from build123d import *

# Parameters (mm, degrees)
F0_R     = 74.8
F0_R_2   = 3.5
F0_R_3   = 26
F1_DEPTH = 7.9
F2_DEPTH = 7.9
F3_R     = 66.1
F3_R_2   = 3.5
F3_R_3   = 26
F4_DEPTH = 2
F8_DEPTH = 5.9
F9_DEPTH = 2


# Not quite as in the source:
# - a feature names something its author has since deleted; it is built from what else it names


with BuildPart() as f1:
    # F0 (on Front) → F1 (new body)
    with BuildSketch(Plane.XZ):
        Circle(F0_R)
        with BuildLine():
            ThreePointArc((-23.816128087, -54.7983078474), (-42.2496301759, -42.2496301759), (-54.7983078474, -23.816128087))
            ThreePointArc((-54.7983078474, -23.816128087), (-54.50218665, -19.353932752), (-51.1097752784, -22.2677652896))
            ThreePointArc((-51.1097752784, -22.2677652896), (-39.4212030512, -39.4212030512), (-22.2677652896, -51.1097752784))
            ThreePointArc((-22.2677652896, -51.1097752784), (-19.353932752, -54.50218665), (-23.816128087, -54.7983078474))
        make_face(mode=Mode.SUBTRACT)
        with Locations((0, -42.7)):
            Circle(F0_R_2, mode=Mode.SUBTRACT)
        Circle(F0_R_3, mode=Mode.SUBTRACT)
        with BuildLine():
            ThreePointArc((54.7983078474, -23.816128087), (42.2496301759, -42.2496301759), (23.816128087, -54.7983078474))
            ThreePointArc((23.816128087, -54.7983078474), (19.353932752, -54.50218665), (22.2677652896, -51.1097752784))
            ThreePointArc((22.2677652896, -51.1097752784), (39.4212030512, -39.4212030512), (51.1097752784, -22.2677652896))
            ThreePointArc((51.1097752784, -22.2677652896), (54.50218665, -19.353932752), (54.7983078474, -23.816128087))
        make_face(mode=Mode.SUBTRACT)
        with BuildLine():
            ThreePointArc((-54.7983078474, 23.816128087), (-42.2496301759, 42.2496301759), (-23.816128087, 54.7983078474))
            ThreePointArc((-23.816128087, 54.7983078474), (-19.353932752, 54.50218665), (-22.2677652896, 51.1097752784))
            ThreePointArc((-22.2677652896, 51.1097752784), (-39.4212030512, 39.4212030512), (-51.1097752784, 22.2677652896))
            ThreePointArc((-51.1097752784, 22.2677652896), (-54.50218665, 19.353932752), (-54.7983078474, 23.816128087))
        make_face(mode=Mode.SUBTRACT)
        with Locations((0, 42.7)):
            Circle(F0_R_2, mode=Mode.SUBTRACT)
        with BuildLine():
            ThreePointArc((54.7983078474, 23.816128087), (54.50218665, 19.353932752), (51.1097752784, 22.2677652896))
            ThreePointArc((51.1097752784, 22.2677652896), (39.4212030512, 39.4212030512), (22.2677652896, 51.1097752784))
            ThreePointArc((22.2677652896, 51.1097752784), (19.353932752, 54.50218665), (23.816128087, 54.7983078474))
            ThreePointArc((23.816128087, 54.7983078474), (42.2496301759, 42.2496301759), (54.7983078474, 23.816128087))
        make_face(mode=Mode.SUBTRACT)
        Circle(F0_R_3)
    extrude(amount=-F1_DEPTH)

    # F0 (on Front) → F2 (cut)
    with BuildSketch(Plane.XZ):
        Circle(F0_R_3)
    extrude(amount=-F2_DEPTH, mode=Mode.SUBTRACT)

    # F3 (on face) → F4 (cut)
    with BuildSketch(Plane.XZ):
        Circle(F3_R)
        with BuildLine():
            ThreePointArc((-22.2677652896, -51.1097752784), (-19.353932752, -54.50218665), (-23.816128087, -54.7983078474))
            ThreePointArc((-23.816128087, -54.7983078474), (-42.2496301759, -42.2496301759), (-54.7983078474, -23.816128087))
            ThreePointArc((-54.7983078474, -23.816128087), (-54.50218665, -19.353932752), (-51.1097752784, -22.2677652896))
            ThreePointArc((-51.1097752784, -22.2677652896), (-39.4212030512, -39.4212030512), (-22.2677652896, -51.1097752784))
        make_face(mode=Mode.SUBTRACT)
        with Locations((0, -42.7)):
            Circle(F3_R_2, mode=Mode.SUBTRACT)
        Circle(F3_R_3, mode=Mode.SUBTRACT)
        with BuildLine():
            ThreePointArc((51.1097752784, -22.2677652896), (54.50218665, -19.353932752), (54.7983078474, -23.816128087))
            ThreePointArc((54.7983078474, -23.816128087), (42.2496301759, -42.2496301759), (23.816128087, -54.7983078474))
            ThreePointArc((23.816128087, -54.7983078474), (19.353932752, -54.50218665), (22.2677652896, -51.1097752784))
            ThreePointArc((22.2677652896, -51.1097752784), (39.4212030512, -39.4212030512), (51.1097752784, -22.2677652896))
        make_face(mode=Mode.SUBTRACT)
        with BuildLine():
            ThreePointArc((-51.1097752784, 22.2677652896), (-54.50218665, 19.353932752), (-54.7983078474, 23.816128087))
            ThreePointArc((-54.7983078474, 23.816128087), (-42.2496301759, 42.2496301759), (-23.816128087, 54.7983078474))
            ThreePointArc((-23.816128087, 54.7983078474), (-19.353932752, 54.50218665), (-22.2677652896, 51.1097752784))
            ThreePointArc((-22.2677652896, 51.1097752784), (-39.4212030512, 39.4212030512), (-51.1097752784, 22.2677652896))
        make_face(mode=Mode.SUBTRACT)
        with Locations((0, 42.7)):
            Circle(F3_R_2, mode=Mode.SUBTRACT)
        with BuildLine():
            ThreePointArc((23.816128087, 54.7983078474), (42.2496301759, 42.2496301759), (54.7983078474, 23.816128087))
            ThreePointArc((54.7983078474, 23.816128087), (54.50218665, 19.353932752), (51.1097752784, 22.2677652896))
            ThreePointArc((51.1097752784, 22.2677652896), (39.4212030512, 39.4212030512), (22.2677652896, 51.1097752784))
            ThreePointArc((22.2677652896, 51.1097752784), (19.353932752, 54.50218665), (23.816128087, 54.7983078474))
        make_face(mode=Mode.SUBTRACT)
    extrude(amount=-F4_DEPTH, mode=Mode.SUBTRACT)

    # F5 (on Right) → F6 (revolve, cut)
    with BuildSketch(Plane.YZ):
        Polygon((-1.7160152132, 0), (2, 0), (2, 66.1), (-1.7160152132, 74.0690203414), align=None)
    revolve(axis=Axis((0, 0.1419923934, 0), (0, 1, 0)), mode=Mode.SUBTRACT)

    # F7 (on face) → F8 (cut)
    with BuildSketch(Plane.XZ.offset(-2)):
        Polygon((-6, 70.3), (-6, 66.5), (6, 66.5), (6, 70.3), (12.4951375847, 76.7951375847), (-12.3430622144, 76.6430622144), align=None)
        Polygon((-66.5, 6), (-70.3, 6), (-76.7951375847, 12.4951375847), (-76.6430622144, -12.3430622144), (-70.3, -6), (-66.5, -6), align=None)
        Polygon((-6, -66.5), (-6, -70.3), (-12.4951375847, -76.7951375847), (12.3430622144, -76.6430622144), (6, -70.3), (6, -66.5), align=None)
        Polygon((66.5, -6), (70.3, -6), (76.7951375847, -12.4951375847), (76.6430622144, 12.3430622144), (70.3, 6), (66.5, 6), align=None)
    extrude(amount=-F8_DEPTH, mode=Mode.SUBTRACT)

    # F9 (cut): faces of the model
    f9_faces = [f1.faces().sort_by_distance(p)[0] for p in [
        (0, 2, 70.9549233508),
        (0, 2, -70.9549233508),
        (-70.9549233508, 2, 0),
        (70.9549233508, 2, 0),
    ]]
    extrude(f9_faces, amount=-F9_DEPTH, mode=Mode.SUBTRACT)


solid = f1.part
Work out the finished part from the listing and answer in its coordinate system (mm). A direction names the side the tool comes from. Coordinates: 2 decimals unless noted, no trailing zeros. Order: outer loops, then holes, each group sorted by start corner. A loop starts at its lowest first (then second) coordinate and runs counter-clockwise, first axis right, second up. Notation, with made-up numbers: (32, -6) - (83, -6) arc R24 cw to (83, 5) - close; hole circle Ø9 at (-4.5, -12.5). An arc over 180 degrees is marked (long way). Put each result on its own line as item: value. Start each with the question number.
1) Find section C-C (y = 4). State how many separate pieces and enclosed holes the cut face has, plus the area to 3 significant figures.
2) Flat-ended cylindrical pins translate along their axes: pin 1 (4 mm diameter, centred on x = -51.5, y = 5.5, fed in from +Z); pin 2 (1.9 mm diameter, centred on x = -1, y = 5, fed in from -Z); pin 3 (4.5 mm diameter, centred on x = 53.53, z = -21.66, fed in from +Y); pin 4 (3 mm diameter, centred on x = -28.5, z = -7, fed in from -Y). Find the tip coordinate at first contact, or state that the pin passes through.
3) For a pull along Z with two mould halves and no side action, classify faces 4 (the cylindrical face through (52.41, 3.89, -53.37)), 5 (the cylindrical face through (-39.63, 4.91, -39.21)), 6 (the cylindrical face through (-52.41, 3.89, 53.37)) as released by +Z, released by -Z, zero draft, split by the parting line, or undercut.
4) Find section A-A (x = 0). Give the vertices of the cut face in (y, z), plus the area to 3 significant figures.
5) Find section B-B (z = 0). Give the vertices of the cut face in (x, y).
6) For faces 1 (the flat face through (6, 4, -68)), 2 (the cylindrical face through (42, 4.9, 42.5)), 3 (the flat face through (72.2, 4, -7.9)), determine the directions among +Z, -Z, +X, -X, +Y, -Y from which every point of the face is accessible in a straight line to the end or side of a thin tool.
7) Find the intervals of material crossed by line 1 (Z direction, x = 0, y = 3.55); line 2 (Z direction, x = 24, y = 3.5); line 3 (X direction, y = 3.5, z = 50), in increasing order. Write a range as from..to.
Results list:
1. separate pieces: 1
1. enclosed holes: 7
1. area: 14,100 mm^2
2. pin 1: stops at z = 56.08
2. pin 2: stops at z = -66.5
2. pin 3: passes through
2. pin 4: stops at y = 2
3. face 4: released by -Z
3. face 5: undercut
3. face 6: released by +Z
4. outline: (1.81, -66.5) - (7.9, -66.5) - (7.9, -46.2) - (2, -46.2) - (2, -66.1) - close; (1.81, 66.5) - (2, 66.1) - (2, 46.2) - (7.9, 46.2) - (7.9, 66.5) - close; (2, -39.2) - (7.9, -39.2) - (7.9, -26) - (2, -26) - close; (2, 26) - (7.9, 26) - (7.9, 39.2) - (2, 39.2) - close
4. area: 395 mm^2
5. outline: (-66.5, 1.81) - (-66.1, 2) - (-26, 2) - (-26, 7.9) - (-66.5, 7.9) - close; (26, 2) - (66.1, 2) - (66.5, 1.81) - (66.5, 7.9) - (26, 7.9) - close
6. face 1: -Z, +Y, -Y
6. face 2: +Y, -Y
6. face 3: +X, +Y, -Y
7. line 1: z = -66.5..-46.2, -39.2..-26, 26..39.2, 46.2..66.5
7. line 2: z = -70.85..-54.72, -50.32..-10, 10..50.32, 54.72..70.85
7. line 3: x = -55.63..-32.71, -24.66..24.66, 32.71..55.63
